Autodesk Inventor part; units mm, degrees
ref_plane "YZ Plane" through (0, 0, 0) normal (1, 0, 0) x (0, 1, 0)
ref_plane "XZ Plane" through (0, 0, 0) normal (0, 1, 0) x (-1, 0, 0)
ref_plane "XY Plane" through (0, 0, 0) normal (0, 0, 1) x (1, 0, 0)
sketch "Sketch1" plane through (0, 0, 0) normal (0, 1, 0) x (-1, 0, 0)
  circle A0 centre (0, 0) radius 14.8
  circle A1 centre (0, 0) radius 18.6876
  dimension "d0" = 29.6
extrude "Extrusion1" add sketch "Sketch1" along normal blind 5
sketch "Sketch2" plane through (0, 5, 0) normal (0, 1, 0) x (1, 0, 0)
  line L0 (0, 0) -> (0, 26)
  line L1 (0, 26) -> (-26, 26)
  line L2 (-26, 26) -> (-26, -26)
  line L3 (-26, -26) -> (26, -26)
  line L4 (26, -26) -> (26, 26)
  line L5 (26, 26) -> (-26, 26)
  line L6 (-26, 26) -> (-26, -26)
  dimension "d3" = 26
  dimension "d4" = 26
  dimension "d5" = 52
  dimension "d6" = 52
extrude "Extrusion2" add sketch "Sketch2" along normal blind 7
sketch "Sketch3" plane through (0, 5, 0) normal (0, -1, 0) x (1, 0, 0)
  circle A0 centre (9.5, 0) radius 1.8
  circle A1 centre (-9.5, 0) radius 1.8
  circle A2 centre (0, -8) radius 1.8
  circle A3 centre (0, 8) radius 1.8
  circle A4 centre (0, 0) radius 3
  dimension "d11" = 3.6
  dimension "d12" = 3.6
  dimension "d13" = 3.6
  dimension "d14" = 3.6
  dimension "d15" = 6
extrude "Extrusion3" cut sketch "Sketch3" against normal blind 15
sketch "Sketch4" plane through (26, 5, 26) normal (1, 0, 0) x (0, 0, -1)
  line L0 (52, 0) -> (0, 0)
  line L1 (26, 0) -> (26, 1)
  circle A0 centre (26, 1) radius 5.8
  circle A1 centre (26, 1) radius 11.4632
  point P0 (26, -5)
  dimension "d18" = 1
  dimension "d19" = 11.6
extrude "Extrusion4" add sketch "Sketch4" along normal blind 19.5 and the other way blind 10.5 contours A1 L0 A0 | L0 A0 A1
sketch "Sketch5" plane through (45.5, 6, 0) normal (1, 0, 0) x (0, 0, -1)
  circle A0 centre (0, 0) radius 5.8
  circle A1 centre (0, 0) radius 5.8
  point P0 (0, -6)
extrude "Extrusion5" cut sketch "Sketch5" against normal blind 32
sketch "Sketch6" plane through (0, 12, 0) normal (0, 1, 0) x (1, 0, 0)
  line L0 (0, 0) -> (0, 22.5)
  line L1 (0, 22.5) -> (-22.5, 22.5)
  line L2 (-22.5, 22.5) -> (-22.5, -22.5)
  line L3 (-22.5, -22.5) -> (22.5, -22.5)
  line L4 (22.5, -22.5) -> (22.5, 22.5)
  circle A0 centre (-22.5, 22.5) radius 1.8
  circle A1 centre (22.5, 22.5) radius 1.8
  circle A2 centre (-22.5, -22.5) radius 1.8
  circle A3 centre (22.5, -22.5) radius 1.8
  dimension "d26" = 22.5
  dimension "d27" = 22.5
  dimension "d28" = 45
  dimension "d29" = 45
  dimension "d30" = 3.6
  dimension "d31" = 3.6
  dimension "d32" = 3.6
  dimension "d33" = 3.6
extrude "Extrusion6" cut sketch "Sketch6" against normal blind 32
properties part number "NewGimbalPart4" material "Brass, Soft Yellow, Welded"
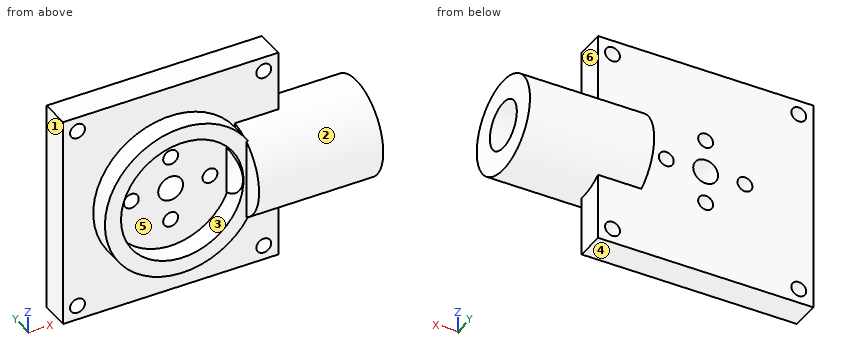
Design review of the part built by this model. Coordinates are the model's own, in mm. Face numbers are marked on the shaded views. A direction names the side the tool comes from. Give positions to 0.01 mm unless a question says otherwise; leave off trailing zeros. Order: outer loops, then holes, each group sorted by start corner. A loop starts at its lowest first (then second) coordinate and runs counter-clockwise, first axis right, second up. Notation, with made-up numbers: (-16, 45.25) - (-7, 45.25) arc R24 ccw to (-7, 63.25) - close; hole circle Ø5 at (32, 30). An arc over 180 degrees is marked (long way). Write item = value, one per line. Start each with the question number.
Q1. Clearance check with flat-ended pins moving along their axes: pin 1 Ø4 at (x, z) = (-18.5, 17) entering from -Y; pin 2 Ø6 at (y, z) = (0.5, 17) entering from -X; pin 3 Ø1.1 at (y, z) = (3.5, 10.5) entering from -X. State where each tip first meets the part, or that it passes through.
Q2. To check wall thickness, follow L1, parallel to Z at x = 0, y = 9.5; L2, parallel to Z at x = 22.5, y = 6.5; L3, parallel to Z at x = -9.5, y = 9. State the ranges of each line that lie inside material, in increasing order. Write a range as from..to.
Q3. Tool access review of the marked faces 1, 2 and 3: name each direction out of +Z, -Z, +X, -X, +Y, -Y from which nothing blocks a thin tool from reaching the whole face with its end or side.
Q4. We need section D-D on x = -22.5. State the section outline as (y, z) points, plus the area to 3 significant figures.
Q5. Mouldability with a two-part tool opening along X and no side actions: class the marked faces 4, 5 and 6 as released by +X, released by -X, zero draft, split by the parting line, or undercut.
Q6. We need section B-B on x = 0. State the section outline as (y, z) points, plus the area to 3 significant figures.
Q7. We need section C-C on x = 21.5. State the section outline as (y, z) points.
Q8. We need section A-A on z = -22.5. State the section outline as (x, y) points.
Working result:
q1.pin_1 = 5
q1.pin_2 = -12.38
q1.pin_3 = -15.82
q2.L1 = -26..-9.8, -6.2..-3, 3..6.2, 9.8..26
q2.L2 = -26..-24.3, -20.7..-5.78, 5.78..20.7, 24.3..26
q2.L3 = -26..-1.8, 1.8..26
q3.face_1 = +Z, -Z, -X, +Y, -Y
q3.face_2 = +X
q3.face_3 = -Y
q4.outline = (5, -26) - (12, -26) - (12, -24.3) - (5, -24.3) - close; (5, -20.7) - (12, -20.7) - (12, 20.7) - (5, 20.7) - close; (5, 24.3) - (12, 24.3) - (12, 26) - (5, 26) - close
q4.area = 314 mm²
q5.face_4 = zero draft
q5.face_5 = undercut
q5.face_6 = released by +X
q6.outline = (0, -18.69) - (5, -18.69) - (5, -26) - (12, -26) - (12, -9.8) - (5, -9.8) - (5, -14.8) - (0, -14.8) - close; (0, 14.8) - (5, 14.8) - (5, 9.8) - (12, 9.8) - (12, 26) - (5, 26) - (5, 18.69) - (0, 18.69) - close; (5, -6.2) - (12, -6.2) - (12, -3) - (5, -3) - close; (5, 3) - (12, 3) - (12, 6.2) - (5, 6.2) - close
q6.area = 310 mm²
q7.outline = (5, -26) - (12, -26) - (12, -24) - (5, -24) - close; (5, -21) - (12, -21) - (12, -9.77) arc R11.46 ccw to (12, 9.77) - (12, 21) - (5, 21) - (5, 11.42) arc R11.46 ccw to (5, -11.42) - close; (5, 24) - (12, 24) - (12, 26) - (5, 26) - close; hole circle Ø11.6 at (6, 0)
q8.outline = (-26, 5) - (-24.3, 5) - (-24.3, 12) - (-26, 12) - close; (-20.7, 5) - (20.7, 5) - (20.7, 12) - (-20.7, 12) - close; (24.3, 5) - (26, 5) - (26, 12) - (24.3, 12) - close
